Could you check a few things on this model? Use its own coordinates, in mm. Coordinates: 2 decimals unless noted, no trailing zeros. Write each loop counter-clockwise with the first axis right and the second up, starting at its lowest first coordinate (ties: lowest second). Pieces come first, ordered by that corner, then holes. Notation, with made-up numbers: (61.25, 21.25) - (80.25, 21.25) arc R10 cw to (80.25, 39.25) - close; hole circle Ø5 at (-20, -12). An arc over 180 degrees is marked (long way). Answer as a JSON object with one key per item and string values. Group by question number.
1) If we section it at B-B (x = 270): Write out the boundary of the cut face in (y, z), plus the area to 3 significant figures.
2) Will these pins go through, and if not, where does the flat tip stop? pin 1 Ø2 at (y, z) = (338.5, 14.5) entering from -X; pin 2 Ø3 at (x, z) = (326.25, 9.52) entering from +Y; pin 3 Ø3 at (y, z) = (285, 11.5) entering from -X.
3) If we section it at A-A (x = 114): Write out the boundary of the cut face in (y, z).
4) If we section it at C-C (y = 276.5): Write out the boundary of the cut face in (x, z).
5) If we section it at D-D (y = 212): Write out the boundary of the cut face in (x, z), plus the area to 3 significant figures.
6) Please list where these lines run through material, in increasing order: line 1 along Y through (x, z) = (134, 8.5); line 2 along X through (y, z) = (380, 17.25); line 3 along X through (y, z) = (170, 1.5).
```python
from build123d import *

# Parameters (mm, degrees)
MODEL_R             = 2.5146
BOSS_EXTRUDE1_DEPTH = 19.05
CUT_EXTRUDE1_REACH  = 439.02
SKETCH2_R           = 2.5527
CUT_EXTRUDE2_REACH  = 439.02
SKETCH3_R           = 2.5527


with BuildPart() as part:
    # Model → Boss-Extrude1 (new body)
    with BuildSketch(Plane.XY):
        with BuildLine():
            Line((332.980192528, 413.072749717), (91.680192525, 413.072749717))
            ThreePointArc((91.680192525, 413.072749717), (82.699936404, 409.353005838), (78.980192525, 400.372749717))
            Line((78.980192525, 400.372749717), (78.980192525, 374.972749717))
            ThreePointArc((78.980192525, 374.972749717), (82.699936404, 365.992493596), (91.680192525, 362.272749717))
            Line((91.680192525, 362.272749717), (136.130192525, 362.272749717))
            ThreePointArc((136.130192525, 362.272749717), (154.090704768, 354.833261959), (161.530192525, 336.872749717))
            Line((161.530192525, 336.872749717), (161.530192525, 222.572749717))
            ThreePointArc((161.530192525, 222.572749717), (154.090704768, 204.612237475), (136.130192525, 197.172749717))
            Line((136.130192525, 197.172749717), (91.680192525, 197.172749717))
            ThreePointArc((91.680192525, 197.172749717), (82.699936404, 193.453005838), (78.980192525, 184.472749717))
            Line((78.980192525, 184.472749717), (78.980192525, 159.072749717))
            ThreePointArc((78.980192525, 159.072749717), (82.699936404, 150.092493596), (91.680192525, 146.372749717))
            Line((91.680192525, 146.372749717), (332.980192528, 146.372749717))
            ThreePointArc((332.980192528, 146.372749717), (341.960448649, 150.092493596), (345.680192528, 159.072749717))
            Line((345.680192528, 159.072749717), (345.680192528, 184.472749717))
            ThreePointArc((345.680192528, 184.472749717), (341.960448648, 193.453005839), (332.980192525, 197.172749717))
            Line((332.980192525, 197.172749717), (288.530192525, 197.172749717))
            ThreePointArc((288.530192525, 197.172749717), (270.569680283, 204.612237475), (263.130192525, 222.572749717))
            Line((263.130192525, 222.572749717), (263.130192525, 336.872749717))
            ThreePointArc((263.130192525, 336.872749717), (270.569680284, 354.83326196), (288.530192528, 362.272749717))
            Line((288.530192528, 362.272749717), (332.980192528, 362.272749717))
            ThreePointArc((332.980192528, 362.272749717), (341.960448649, 365.992493596), (345.680192528, 374.972749717))
            Line((345.680192528, 374.972749717), (345.680192528, 400.372749717))
            ThreePointArc((345.680192528, 400.372749717), (341.960448649, 409.353005838), (332.980192528, 413.072749717))
        make_face()
        with Locations(Location((123.430192525, 387.672749717, 0), (0, 0, 180))):
            Circle(MODEL_R, mode=Mode.SUBTRACT)
        with Locations(Location((301.230192525, 387.672749717, 0), (0, 0, 180))):
            Circle(MODEL_R, mode=Mode.SUBTRACT)
        with Locations(Location((123.430192525, 171.772749717, 0), (0, 0, 180))):
            Circle(MODEL_R, mode=Mode.SUBTRACT)
        with Locations(Location((301.230192525, 171.772749717, 0), (0, 0, 180))):
            Circle(MODEL_R, mode=Mode.SUBTRACT)
        with BuildLine():
            ThreePointArc((330.402277638, 163.888053974), (331.440317525, 171.772749717), (330.402277638, 179.657445459))
            ThreePointArc((330.402277638, 179.657445459), (324.511101714, 183.058717465), (321.109829708, 177.167541541))
            ThreePointArc((321.109829708, 177.167541541), (321.820067525, 171.772749717), (321.109829708, 166.377957893))
            ThreePointArc((321.109829708, 166.377957893), (324.511101714, 160.486781969), (330.402277638, 163.888053974))
        make_face(mode=Mode.SUBTRACT)
        with BuildLine():
            ThreePointArc((103.550555343, 177.167541541), (102.840317525, 171.772749717), (103.550555343, 166.377957893))
            ThreePointArc((103.550555343, 166.377957893), (100.149283337, 160.486781969), (94.258107413, 163.888053974))
            ThreePointArc((94.258107413, 163.888053974), (93.220067525, 171.772749717), (94.258107413, 179.657445459))
            ThreePointArc((94.258107413, 179.657445459), (100.149283337, 183.058717465), (103.550555343, 177.167541541))
        make_face(mode=Mode.SUBTRACT)
        with BuildLine():
            ThreePointArc((321.109829708, 382.277957893), (321.820067525, 387.672749717), (321.109829708, 393.067541541))
            ThreePointArc((321.109829708, 393.067541541), (324.511101714, 398.958717465), (330.402277638, 395.557445459))
            ThreePointArc((330.402277638, 395.557445459), (331.440317525, 387.672749717), (330.402277638, 379.788053974))
            ThreePointArc((330.402277638, 379.788053974), (324.511101714, 376.386781969), (321.109829708, 382.277957893))
        make_face(mode=Mode.SUBTRACT)
        with BuildLine():
            ThreePointArc((94.258107413, 395.557445459), (93.220067525, 387.672749717), (94.258107413, 379.788053974))
            ThreePointArc((94.258107413, 379.788053974), (100.149283337, 376.386781969), (103.550555343, 382.277957893))
            ThreePointArc((103.550555343, 382.277957893), (102.840317525, 387.672749717), (103.550555343, 393.067541541))
            ThreePointArc((103.550555343, 393.067541541), (100.149283337, 398.958717465), (94.258107413, 395.557445459))
        make_face(mode=Mode.SUBTRACT)
    extrude(amount=BOSS_EXTRUDE1_DEPTH)

    # Sketch2 → Cut-Extrude1 (cut, up to next)
    with BuildSketch(Plane(origin=(0, 413.072749717, 0), x_dir=(1, 0, 0), z_dir=(0, 1, 0)), mode=Mode.PRIVATE) as cut_extrude1_sk1:
        with Locations(Location((98.411192525, -9.525, 0), (0, 0, 180))):
            Circle(SKETCH2_R)
    cut_extrude1_tool1 = extrude(cut_extrude1_sk1.sketch, amount=-CUT_EXTRUDE1_REACH, mode=Mode.PRIVATE) & part.part
    # Sketch2 → Cut-Extrude1 (cut, up to next)
    with BuildSketch(Plane(origin=(0, 413.072749717, 0), x_dir=(1, 0, 0), z_dir=(0, 1, 0)), mode=Mode.PRIVATE) as cut_extrude1_sk2:
        with Locations(Location((326.249192528, -9.525, 0), (0, 0, 180))):
            Circle(SKETCH2_R)
    cut_extrude1_tool2 = extrude(cut_extrude1_sk2.sketch, amount=-CUT_EXTRUDE1_REACH, mode=Mode.PRIVATE) & part.part
    add(cut_extrude1_tool1.solids().sort_by_distance((98.411193, 413.07275, 9.525))[0], mode=Mode.SUBTRACT)
    add(cut_extrude1_tool2.solids().sort_by_distance((326.249193, 413.07275, 9.525))[0], mode=Mode.SUBTRACT)

    # Sketch3 → Cut-Extrude2 (cut, up to next)
    with BuildSketch(Plane.XZ.offset(-146.372749717), mode=Mode.PRIVATE) as cut_extrude2_sk1:
        with Locations(Location((98.411192525, 9.525, 0), (0, 0, 180))):
            Circle(SKETCH3_R)
    cut_extrude2_tool1 = extrude(cut_extrude2_sk1.sketch, amount=-CUT_EXTRUDE2_REACH, mode=Mode.PRIVATE) & part.part
    # Sketch3 → Cut-Extrude2 (cut, up to next)
    with BuildSketch(Plane.XZ.offset(-146.372749717), mode=Mode.PRIVATE) as cut_extrude2_sk2:
        with Locations(Location((326.249192528, 9.525, 0), (0, 0, 180))):
            Circle(SKETCH3_R)
    cut_extrude2_tool2 = extrude(cut_extrude2_sk2.sketch, amount=-CUT_EXTRUDE2_REACH, mode=Mode.PRIVATE) & part.part
    add(cut_extrude2_tool1.solids().sort_by_distance((98.411193, 146.37275, 9.525))[0], mode=Mode.SUBTRACT)
    add(cut_extrude2_tool2.solids().sort_by_distance((326.249193, 146.37275, 9.525))[0], mode=Mode.SUBTRACT)


solid = part.part
```
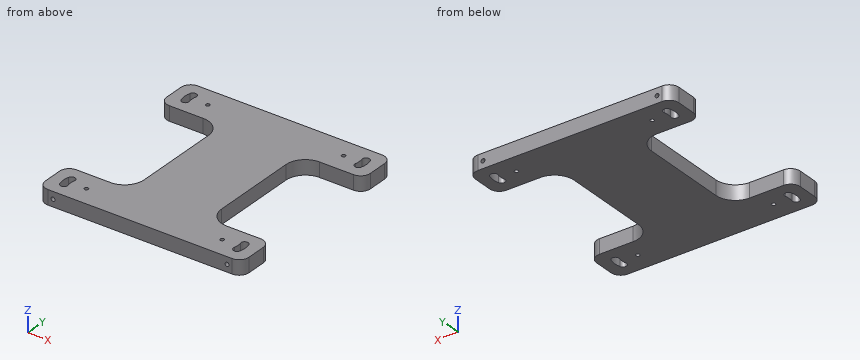
Here are the results:
{
 "1": {"outline": "(146.37, 0) - (205.2, 0) - (205.2, 19.05) - (146.37, 19.05) - close; (354.24, 0) - (413.07, 0) - (413.07, 19.05) - (354.24, 19.05) - close", "area": "2,240 mm²"},
 "2": {"pin 1": "stops at x = 161.39", "pin 2": "stops at y = 376.66", "pin 3": "stops at x = 161.53"},
 "3": {"outline": "(146.37, 0) - (197.17, 0) - (197.17, 19.05) - (146.37, 19.05) - close; (362.27, 0) - (413.07, 0) - (413.07, 19.05) - (362.27, 19.05) - close"},
 "4": {"outline": "(161.53, 0) - (263.13, 0) - (263.13, 19.05) - (161.53, 19.05) - close"},
 "5": {"outline": "(159.23, 0) - (265.44, 0) - (265.44, 19.05) - (159.23, 19.05) - close", "area": "2,020 mm²"},
 "6": {"line 1": "y = 146.37 to 197.17, 362.27 to 413.07", "line 2": "x = 78.98 to 94.2, 103.6 to 321.06, 330.46 to 345.68", "line 3": "x = 78.98 to 93.27, 102.92 to 121.65, 125.21 to 299.45, 303.01 to 321.74, 331.39 to 345.68"}
}
